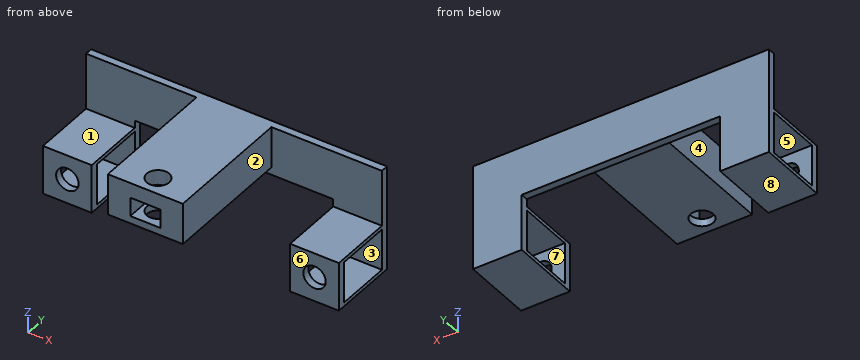
from build123d import *

# Parameters (mm, degrees)
SKETCH_2_W               = 13
SKETCH_2_H               = 13
SKETCH_2_R               = 3
EXTRUDE_1_DEPTH          = 2
EXTRUDE_1_2_DEPTH        = 2
SKETCH_3_W               = 13
SKETCH_3_H               = 1
EXTRUDE_2_DEPTH          = 15
SKETCH_4_W               = 13
SKETCH_4_H               = 12
SKETCH_4_H_2             = 1
SKETCH_4_W_2             = 53
SKETCH_4_H_3             = 13
EXTRUDE_3_DEPTH          = 2
SKETCH_5_W               = 20
SKETCH_5_H               = 11
EXTRUDE_4_DEPTH          = 37
CUT_EXTRUDE_1_DEPTH      = 84.246621553
CUT_EXTRUDE_1_DEPTH_BACK = 84.246621553
SKETCH_6_R               = 3
SKETCH_7_W               = 8
SKETCH_7_H               = 5
CUT_EXTRUDE_2_DEPTH      = 17
SKETCH_8_W               = 20
SKETCH_8_H               = 11
CUT_EXTRUDE_3_DEPTH      = 2


with BuildPart() as part:
    # Sketch 2 → Extrude 1 (new body)
    with BuildSketch(Plane(origin=(0, 0, 0), x_dir=(1, 0, 0), z_dir=(0, 1, 0))):
        with Locations((6.5, 6.5)):
            Rectangle(SKETCH_2_W, SKETCH_2_H)
        with Locations(Location((6.5, 6.5, 0), (0, 0, 270))):
            Circle(SKETCH_2_R, mode=Mode.SUBTRACT)
    extrude(amount=EXTRUDE_1_DEPTH)



with BuildPart() as body_2:
    # Sketch 2 → Extrude 1 2 (new body)
    with BuildSketch(Plane(origin=(0, 0, 0), x_dir=(1, 0, 0), z_dir=(0, 1, 0))):
        with Locations((72.5, 6.5)):
            Rectangle(SKETCH_2_W, SKETCH_2_H)
        with Locations(Location((72.5, 6.5, 0), (0, 0, 90))):
            Circle(SKETCH_2_R, mode=Mode.SUBTRACT)
    extrude(amount=EXTRUDE_1_2_DEPTH)


with BuildPart() as part_1:
    add(part.part)

    add(body_2.part)  # Extrude 2 merges body 2
    # Sketch 3 → Extrude 2 (add)
    with BuildSketch(Plane(origin=(0, 2, 0), x_dir=(1, 0, 0), z_dir=(0, 1, 0))):
        with Locations((6.5, 12.5)):
            Rectangle(SKETCH_3_W, SKETCH_3_H)
        with Locations((6.5, 0.5)):
            Rectangle(SKETCH_3_W, SKETCH_3_H)
        with Locations((72.5, 0.5)):
            Rectangle(SKETCH_3_W, SKETCH_3_H)
        with Locations((72.5, 12.5)):
            Rectangle(SKETCH_3_W, SKETCH_3_H)
    extrude(amount=EXTRUDE_2_DEPTH)

    # Sketch 4 → Extrude 3 (add)
    with BuildSketch(Plane(origin=(0, 17, 0), x_dir=(1, 0, 0), z_dir=(0, 1, 0))):
        Polygon((13, 0), (0, 0), (0, -15), (13, -15), (13, -2), align=None)
        with Locations((6.5, 7)):
            Rectangle(SKETCH_4_W, SKETCH_4_H)
        with Locations((6.5, 0.5)):
            Rectangle(SKETCH_4_W, SKETCH_4_H_2)
        with Locations((39.5, -8.5)):
            Rectangle(SKETCH_4_W_2, SKETCH_4_H_3)
        Polygon((66, -2), (66, -15), (79, -15), (79, 0), (79, 13), (66, 13), (66, 12), (66, 1), (66, 0), align=None)
    extrude(amount=EXTRUDE_3_DEPTH)

    # Sketch 5 → Extrude 4 (add)
    with BuildSketch(Plane.XZ.offset(-17)):
        with Locations((39.5, 9.5)):
            Rectangle(SKETCH_5_W, SKETCH_5_H)
    extrude(amount=EXTRUDE_4_DEPTH)

    # Sketch 6 → Cut-Extrude 1 (cut, two sides: drawn at the far end of the back side and taken through both)
    with BuildSketch(Plane(origin=(0, 0, 4), x_dir=(-1, 0, 0), z_dir=(0, 0, -1)).offset(-CUT_EXTRUDE_1_DEPTH_BACK)):
        with Locations((-39.5, -13)):
            Circle(SKETCH_6_R)
    extrude(amount=CUT_EXTRUDE_1_DEPTH + CUT_EXTRUDE_1_DEPTH_BACK, mode=Mode.SUBTRACT)

    # Sketch 7 → Cut-Extrude 2 (cut)
    with BuildSketch(Plane.XZ.offset(20)):
        with Locations((39.5, 8.5)):
            Rectangle(SKETCH_7_W, SKETCH_7_H)
    extrude(amount=-CUT_EXTRUDE_2_DEPTH, mode=Mode.SUBTRACT)

    # Sketch 8 → Cut-Extrude 3 (cut)
    with BuildSketch(Plane.XZ.offset(20)):
        with Locations((39.5, 9.5)):
            Rectangle(SKETCH_8_W, SKETCH_8_H)
    extrude(amount=-CUT_EXTRUDE_3_DEPTH, mode=Mode.SUBTRACT)


solid = part_1.part
CAD build for the part. Positions are in the model's coordinates, mm. Face numbers are marked on the shaded views. A direction names the side the tool comes from. Give positions to 0.01 mm unless a question says otherwise; leave off trailing zeros. Loops run counter-clockwise (first coordinate to the right, second up) from the corner with the lowest first, then second, coordinate; pieces in that order, holes last. Notation, with made-up numbers: M 89,83 L 112,83 A22 ccw 112,105 Z; hole C 21,49 d2. An arc over 180 degrees is marked long. Write each question's results on one line, items separated by ' | '.
Q1. Band-saw the part on B-B on x = 39.5. Write the cut outline in (y, z), and give its area (3 significant figures).
Geometry check:
outline: M -18,4 L -16,4 L -16,6 L -18,6 Z; M -18,11 L -16,11 L -16,15 L -18,15 Z; M -10,4 L 17,4 L 17,2 L 19,2 L 19,15 L -10,15 L -10,11 L -3,11 L -3,6 L -10,6 Z | area: 300 mm²
Q2. Probe probe 1 along X at (y, z) = (1.3, -6.5); probe 2 along X at (y, z) = (-13, 12.85); probe 3 along Z at (x, y) = (75.5, 4). List the from-to ranges inside material, lowest first.
Geometry check:
probe 1: x = 0 to 3.5, 9.5 to 13, 66 to 69.5, 75.5 to 79 | probe 2: x = 29.5 to 36.5, 42.5 to 49.5 | probe 3: z = -13 to -12, -1 to 0
Q3. Band-saw the part on C-C on z = 6.75. Write the cut outline in (x, y).
Geometry check:
outline: M 0,17 L 29.5,17 L 29.5,-18 L 35.5,-18 L 35.5,-3 L 43.5,-3 L 43.5,-18 L 49.5,-18 L 49.5,17 L 79,17 L 79,19 L 0,19 Z
Q4. Which spindle directions (+Z, -Z, +X, -X, +Y, -Y) get a long thin tool onto all of the face, cutting with end or side? Do the marked faces 1, 2, 3 and 4. Say none if no direction does.
Geometry check:
face 1: +Z, +X, -X, -Y | face 2: +Z, -Z, +X, -Y | face 3: +X, -X | face 4: +Z, -Z, -X, -Y
Q5. Flat gauge pins, fed straight in: P1, Ø10.5, axis at x = 5, y = 7.5, coming from the +Z side; P2, Ø12, axis at y = -2, z = 8.5, coming from the +X side; P3, Ø5.5, axis at y = -10.5, z = 8.5, coming from the -X side; P4, Ø8, axis at x = 61.5, z = -10, coming from the +Y side. Where does each tip first touch, or does it go through?
Geometry check:
P1: stops at z = 0 | P2: stops at x = 49.5 | P3: stops at x = 29.5 | P4: passes through
Q6. Band-saw the part on D-D on y = 3.5. Write the cut outline in (x, z), and give its area (3 significant figures).
Geometry check:
outline: M 0,-13 L 13,-13 L 13,-12 L 0,-12 Z; M 0,-1 L 13,-1 L 13,0 L 0,0 Z; M 29.5,4 L 49.5,4 L 49.5,15 L 29.5,15 Z; M 66,-13 L 79,-13 L 79,-12 L 66,-12 Z; M 66,-1 L 79,-1 L 79,0 L 66,0 Z | area: 272 mm²
Q7. Band-saw the part on A-A on y = -13. Write the cut outline in (x, z).
Geometry check:
outline: M 29.5,4 L 36.5,4 L 36.5,6 L 35.5,6 L 35.5,11 L 36.5,11 L 36.5,15 L 29.5,15 Z; M 42.5,4 L 49.5,4 L 49.5,15 L 42.5,15 L 42.5,11 L 43.5,11 L 43.5,6 L 42.5,6 Z
Q8. Mould opens along Y. For the marked faces 5, 6, 7 and 8 say: pulls with the +Y half, pulls with the -Y half, needs draft (parallel to the pull), parting line crosses it, or undercut.
Geometry check:
face 5: undercut | face 6: pulls with the -Y half | face 7: undercut | face 8: needs draft
